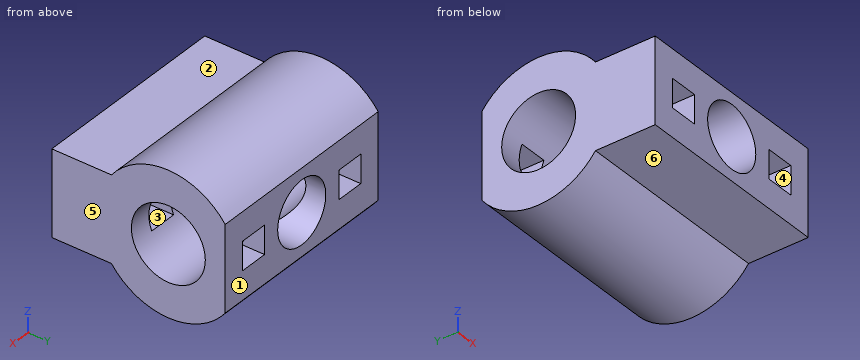
```python
from build123d import *

# Parameters (mm, degrees)
F0_W     = 70
F0_H     = 66
F1_DEPTH = 30
F3_DEPTH = 70
F4_DEPTH = 30
F6_D     = 26
F7_W     = 10
F7_H     = 10
F7_R     = 11
F8_DEPTH = 70


with BuildPart() as f1:
    # F0 (on Top) → F1 (new body)
    with BuildSketch(Plane.XY):
        with Locations((-35.7373842597, 73.1314720511)):
            Rectangle(F0_W, F0_H)
    extrude(amount=F1_DEPTH)

    # F2 (on face) → F3 (join)
    with BuildSketch(Plane(origin=(-70.7373842597, 0, 0), x_dir=(0, -1, 0), z_dir=(-1, 0, 0))):
        with BuildLine():
            Line((-101.1314720511, 30), (-61.1314720511, 30))
            ThreePointArc((-61.1314720511, 30), (-81.1314720511, 40), (-101.1314720511, 30))
        make_face()
        with BuildLine():
            ThreePointArc((-101.1314720511, 0), (-81.1314720511, -10), (-61.1314720511, 0))
            Line((-61.1314720511, 0), (-101.1314720511, 0))
        make_face()
    extrude(amount=-F3_DEPTH)

    # F4 (cut): a face of the model
    f4_faces = [f1.faces().sort_by_distance(p)[0] for p in [
        (-35.7373842597, 103.6314720511, 30),
    ]]
    extrude(f4_faces, amount=-F4_DEPTH, mode=Mode.SUBTRACT)

    # F6 (through all)
    with Locations(Plane(origin=(-70.7373842597, 0, 0), x_dir=(0, -1, 0), z_dir=(-1, 0, 0))):
        with Locations((-81.1314720511, 15)):
            Hole(F6_D / 2)

    # F7 (on face) → F8 (cut)
    with BuildSketch(Plane.XZ.offset(-40.1314720511)):
        with Locations((-57.7373842597, 15)):
            Rectangle(F7_W, F7_H)
        with Locations((-13.7373842597, 15)):
            Rectangle(F7_W, F7_H)
        with Locations((-35.7373842597, 15)):
            Circle(F7_R)
    extrude(amount=-F8_DEPTH, mode=Mode.SUBTRACT)


solid = f1.part
```
Check sheet for the modelled part. Datum: model origin and axes. Units: mm. Face numbers are marked on the shaded views. A direction names the side the tool comes from. Round coordinates to 2 decimals unless told otherwise and drop trailing zeros. Order: outer loops, then holes, each group sorted by start corner. A loop starts at its lowest first (then second) coordinate and runs counter-clockwise, first axis right, second up. Notation, with made-up numbers: (78.25, 21) -> (128.25, 21) arc R28 ccw to (128.25, 47) -> close; hole circle Ø4 at (1, 75.25). An arc over 180 degrees is marked (long way). One line per item, written item: value. Start each with the question number.
Q1. Mould release check, pull along Z, two halves, no side actions. Record for the marked faces 1, 2 and 3: pulls with the +Z half, pulls with the -Z half, needs draft (parallel to the pull), parting line crosses it, or undercut.
Q2. Cross-section at A-A (z = 15). Give the number of separate pieces and of enclosed holes in the cut face, and give its area (3 significant figures).
Q3. Thickness scan on line 1 (X direction, y = 56, z = 15); line 2 (Y direction, x = -48, z = 15); line 3 (X direction, y = 97.5, z = 12). Record the ranges inside material, lowest first.
Q4. Cross-section at C-C (z = 8.5). Record the boundary of the cut face in (x, y).
Q5. Cross-section at D-D (y = 70.5). Record the boundary of the cut face in (x, z), and give its area (3 significant figures).
Q6. Set-up check for the marked faces 4, 5 and 6: record each of +Z, -Z, +X, -X, +Y, -Y from which the full face is reachable in a straight line by a thin tool's end or side.
Q7. Cross-section at B-B (x = -66). Record the boundary of the cut face in (y, z).
Q8. Gauge pin test, flat ends, axial feed: pin 1 Ø4 at (x, y) = (-35, 85) entering from -Z; pin 2 Ø3 at (x, y) = (-9.5, 84) entering from -Z; pin 3 Ø23 at (x, y) = (-30, 52.5) entering from -Z. Record the tip position at first contact, or that the pin passes through.
Completed:
1. face 1: needs draft
1. face 2: pulls with the +Z half
1. face 3: undercut
2. separate pieces: 8
2. enclosed holes: 0
2. area: 980 mm²
3. line 1: x = -70.74 to -62.74, -52.74 to -46.74, -24.74 to -18.74, -8.74 to -0.74
3. line 2: y = 40.13 to 68.13, 94.13 to 101.13
3. line 3: x = -70.74 to -62.74, -52.74 to -46.32, -25.15 to -18.74, -8.74 to -0.74
4. outline: (-70.74, 40.13) -> (-44.61, 40.13) -> (-44.61, 69.87) -> (-70.74, 69.87) -> close; (-70.74, 92.39) -> (-44.61, 92.39) -> (-44.61, 101.13) -> (-70.74, 101.13) -> close; (-26.86, 40.13) -> (-0.74, 40.13) -> (-0.74, 69.87) -> (-26.86, 69.87) -> close; (-26.86, 92.39) -> (-0.74, 92.39) -> (-0.74, 101.13) -> (-26.86, 101.13) -> close
5. outline: (-70.74, -7.63) -> (-0.74, -7.63) -> (-0.74, 7.52) -> (-27.67, 7.52) arc R11 cw to (-43.8, 7.52) -> (-70.74, 7.52) -> close; (-70.74, 22.48) -> (-43.8, 22.48) arc R11 cw to (-27.67, 22.48) -> (-0.74, 22.48) -> (-0.74, 37.63) -> (-70.74, 37.63) -> close
5. area: 2,040 mm²
6. face 4: +Y, -Y
6. face 5: +Z, -Z, +X, +Y, -Y
6. face 6: -Z, +X, -X, -Y
7. outline: (40.13, 0) -> (61.13, 0) arc R25 ccw to (101.13, 0) -> (101.13, 30) arc R25 ccw to (61.13, 30) -> (40.13, 30) -> close; hole circle Ø26 at (81.13, 15)
8. pin 1: stops at z = -9.93
8. pin 2: stops at z = -9.96
8. pin 3: stops at z = -3.21
